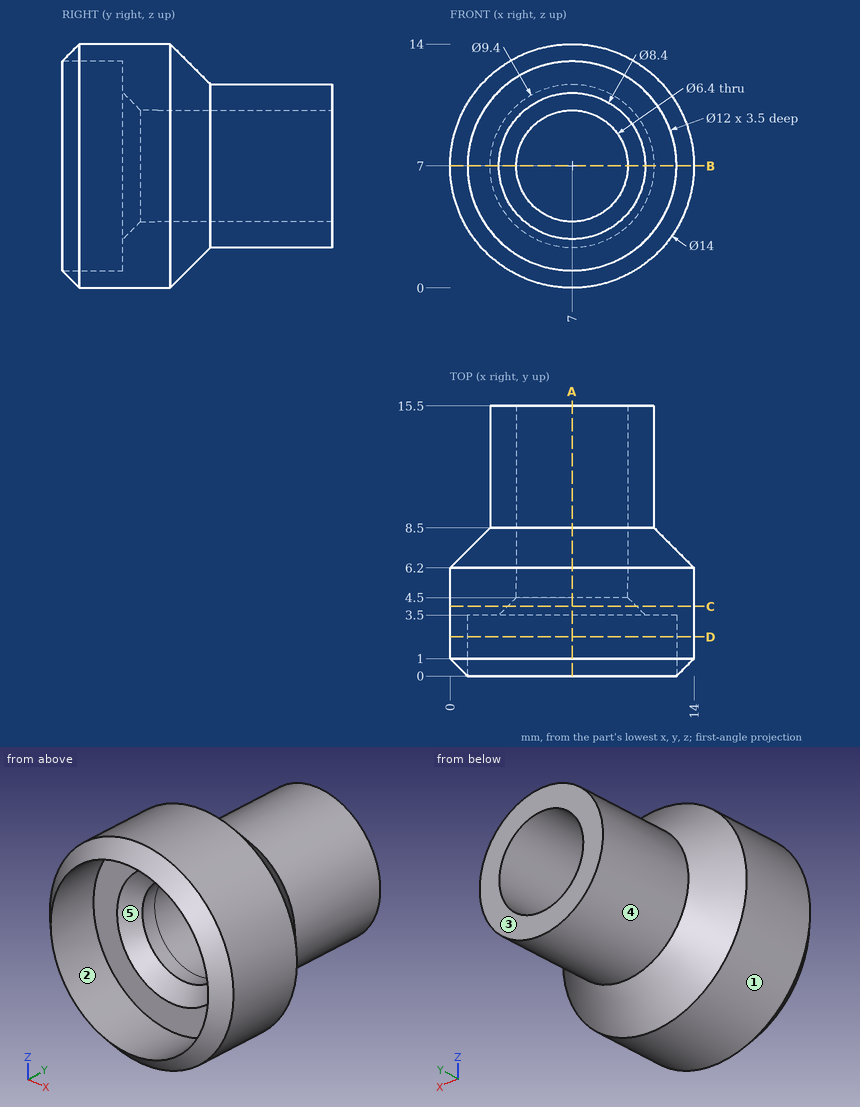
Design review of the part shown in the three views and the two pictorial views. Dimensions are in mm from the part's minimum x, y and z. A direction names the side the tool comes from. Round coordinates to 2 decimals unless told otherwise and drop trailing zeros. Loops run counter-clockwise (first coordinate to the right, second up) from the corner with the lowest first, then second, coordinate; pieces in that order, holes last.
Q1. Insertion check: pin 1 Ø6 at (y, z) = (11.5, 8) entering from -X; pin 2 Ø1 at (y, z) = (2, 12.5) entering from +X; pin 3 Ø1 at (y, z) = (2.5, 8.5) entering from +X; pin 4 Ø4 at (x, y) = (8, 4) entering from -Z. Each pin has a flat end and moves straight along its axis. Give the tip position at first contact, or say it passes through.
Result sheet:
pin 1: stops at x = 2.3
pin 2: stops at x = 11.9
pin 3: stops at x = 13.93
pin 4: stops at z = 0
Q2. To check wall thickness, follow line 1 along X through (y, z) = (5.1, 7); line 2 along Z through (x, y) = (11.75, 2.25); line 3 along Y through (x, z) = (10.5, 4). State the ranges of each line that lie inside material, in increasing order.
Result sheet:
line 1: x = 0 to 3.8, 10.2 to 14
line 2: z = 1.86 to 3.33, 10.67 to 12.14
line 3: y = 3.5 to 15.5
Q3. Add section B-B on z = 7. Write out the cut boundary in (x, y), plus the area to 3 significant figures.
Result sheet:
outline: (0, 1) - (1, 0) - (1, 3.5) - (2.8, 3.5) - (3.8, 4.5) - (3.8, 15.5) - (2.3, 15.5) - (2.3, 8.5) - (0, 6.2) - close; (10.2, 4.5) - (11.2, 3.5) - (13, 3.5) - (13, 0) - (14, 1) - (14, 6.2) - (11.7, 8.5) - (11.7, 15.5) - (10.2, 15.5) - close
area: 58.7 mm2
Q4. Add section A-A on x = 7. Write out the cut boundary in (y, z).
Result sheet:
outline: (0, 1) - (1, 0) - (6.2, 0) - (8.5, 2.3) - (15.5, 2.3) - (15.5, 3.8) - (4.5, 3.8) - (3.5, 2.8) - (3.5, 1) - close; (0, 13) - (3.5, 13) - (3.5, 11.2) - (4.5, 10.2) - (15.5, 10.2) - (15.5, 11.7) - (8.5, 11.7) - (6.2, 14) - (1, 14) - close
Q5. Add section C-C on y = 4. Write out the cut boundary in (x, z), plus the area to 3 significant figures.
Result sheet:
outline: circle Ø14 at (7, 7); hole circle Ø7.4 at (7, 7)
area: 111 mm2
Q6. Mouldability with a two-part tool opening along Z and no side actions: class the marked faces 3, 4 and 5 as +Z half, -Z half, draft (parallel to the pull), parting line (faces both ways), or undercut.
Result sheet:
face 3: draft
face 4: parting line
face 5: undercut
Q7. Machinability: for the marked faces 1 and 2, which of the approach directions +Z, -Z, +X, -X, +Y, -Y give a long, thin tool a straight path to every point of the face, cutting with its end or side? Answer none if there is none.
Result sheet:
face 1: +Y, -Y
face 2: -Y
Q8. Add section D-D on y = 2.25. Write out the cut boundary in (x, z), plus the area to 3 significant figures.
Result sheet:
outline: circle Ø14 at (7, 7); hole circle Ø12 at (7, 7)
area: 40.8 mm2
